Verification items for the finished model (mm, model axes). Face numbers are marked on the shaded views. A direction names the side the tool comes from. Coordinates: 2 decimals unless noted, no trailing zeros. Order: outer loops, then holes, each group sorted by start corner. A loop starts at its lowest first (then second) coordinate and runs counter-clockwise, first axis right, second up. Notation, with made-up numbers: (44.25, -18.5) -> (59.25, -18.5) arc R18 cw to (59.25, -7.5) -> close; hole circle Ø2 at (-33, 35.25). An arc over 180 degrees is marked (long way). Write each question's results on one line, items separated by ' | '. Start each with the question number.
(1) Set-up check for the marked faces 1 and 2: record each of +Z, -Z, +X, -X, +Y, -Y from which the full face is reachable in a straight line by a thin tool's end or side.
(2) Go/stop test with flat-tipped pins: pin 1 (1.5 mm diameter, centred on x = 43, y = -37.5, fed in from -Z); pin 2 (3 mm diameter, centred on y = 41, z = 56, fed in from -X); pin 3 (10 mm diameter, centred on x = 67, y = 9, fed in from -Z). Record where each tip stops, or that it passes through.
(3) Cross-section at A-A on z = 51.5. Enter the section's corners in (x, y), and give its area (3 significant figures).
(4) Thickness scan on probe 1 along Z at (x, y) = (52, -43); probe 2 along X at (y, z) = (-10.5, 26) (3 decimals); probe 3 along X at (y, z) = (5, 39.5). Record the ranges inside material, lowest first. Write a range as [from, to].
(5) Cross-section at B-B on x = 57.5. Enter the section's corners in (y, z).
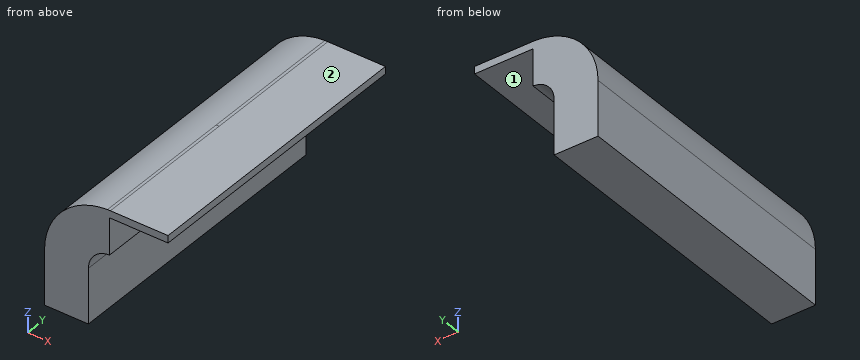
```python
from build123d import *

# Parameters (mm, degrees)
F1_DEPTH = 63.5


with BuildPart() as f1:
    # F0 (on Front) → F1 (new body, symmetric)
    with BuildSketch(Plane.XZ):
        with BuildLine():
            Line((22.225, 33.32649), (22.225, 9.525))
            Line((22.225, 9.525), (41.275, 9.525))
            Line((41.275, 9.525), (41.275, 33.32649))
            ThreePointArc((41.275, 33.32649), (43.941213, 39.945334), (50.450921, 42.86792))
            Line((50.450921, 42.86792), (50.450921, 58.7502))
            Line((50.450921, 58.7502), (75.850921, 58.7502))
            Line((75.850921, 58.7502), (75.850921, 61.9252))
            Line((75.850921, 61.9252), (50.82371, 61.9252))
            add(Edge.make_bspline(
                [(49.53475, 61.896138), (49.965303, 61.908992), (50.394979, 61.918694), (50.82371, 61.9252)],
                knots=[104.865796, 104.865796, 104.865796, 104.865796, 105.962038, 105.962038, 105.962038, 105.962038], degree=3))
            ThreePointArc((49.53475, 61.896138), (30.150674, 53.087861), (22.225, 33.32649))
        make_face()
    extrude(amount=F1_DEPTH, both=True)


solid = f1.part
```
Results are:
1) face 1: -Z, +X, +Y, -Y | face 2: +Z, +X, -X, +Y, -Y
2) pin 1: stops at z = 37.53 | pin 2: stops at x = 31.6 | pin 3: stops at z = 58.75
3) outline: (28.74, -63.5) -> (50.45, -63.5) -> (50.45, 63.5) -> (28.74, 63.5) -> close | area: 2,760 mm2
4) probe 1: z = [58.75, 61.93] | probe 2: x = [22.225, 41.275] | probe 3: x = [22.9, 43.54]
5) outline: (-63.5, 58.75) -> (63.5, 58.75) -> (63.5, 61.93) -> (-63.5, 61.93) -> close
